from build123d import *

# Parameters (mm, degrees)
SKETCH_1_W      = 15.44
SKETCH_1_H      = 15.44
EXTRUDE_1_DEPTH = 17.2
SKETCH_3_R      = 4.9
EXTRUDE_2_DEPTH = 5.5
SKETCH_4_R      = 3.45
EXTRUDE_3_DEPTH = 2


with BuildPart() as part:
    # Эскиз1 → Бобышка-Вытянуть1 (new body)
    with BuildSketch(Plane(origin=(0, 0, 0), x_dir=(1, 0, 0), z_dir=(0, 1, 0))):
        Rectangle(SKETCH_1_W, SKETCH_1_H)
    extrude(amount=EXTRUDE_1_DEPTH)

    # Эскиз2 → section 0 of loft_1
    with BuildSketch(Plane(origin=(0, 29.9, 0), x_dir=(1, 0, 0), z_dir=(0, 1, 0)), mode=Mode.PRIVATE) as loft_1_s0:
        with BuildLine():
            Line((-5.5, 5.5), (5.5, 5.5))
            Line((5.5, 5.5), (5.5, -5.5))
            Line((5.5, -5.5), (-5.5, -5.5))
            Line((-5.5, -5.5), (-5.5, 5.5))
        make_face()
    # loft up to a face of the part (loft_1)
    loft([loft_1_s0.sketch, part.faces().sort_by_distance((0, 17.2, 0))[0]])

    # Эскиз3 → Бобышка-Вытянуть2 (add)
    with BuildSketch(Plane(origin=(0, 29.9, 0), x_dir=(1, 0, 0), z_dir=(0, 1, 0))):
        with Locations(Location((0, 0, 0), (0, 0, 270))):
            Circle(SKETCH_3_R)
    extrude(amount=EXTRUDE_2_DEPTH)

    # Эскиз4 → Бобышка-Вытянуть3 (add)
    with BuildSketch(Plane(origin=(0, 35.4, 0), x_dir=(1, 0, 0), z_dir=(0, 1, 0))):
        with Locations(Location((0, 0, 0), (0, 0, 270))):
            Circle(SKETCH_4_R)
    extrude(amount=EXTRUDE_3_DEPTH)


solid = part.part
Could you check a few things on this model? Use its own coordinates, in mm. A direction names the side the tool comes from. Round coordinates to 2 decimals unless told otherwise and drop trailing zeros.
(1) I'm going to push flat-ended pins straight in: pin 1 (3 mm diameter, centred on x = -2, y = 30, fed in from +Z); pin 2 (5 mm diameter, centred on y = 31.5, z = 2, fed in from +X); pin 3 (1 mm diameter, centred on x = 1, y = 32, fed in from -Z). Where does each tip first touch, or does it pass through?
Response values:
pin 1: stops at z = 5.74
pin 2: stops at x = 5.66
pin 3: stops at z = -4.87
(2) Please list where these lines run through material, in increasing order: line 1 along Y through (x, z) = (1.25, 3.5); line 2 along X through (y, z) = (19, -4.75); line 3 along X through (y, z) = (20, 1.25).
Response values:
line 1: y = 0 to 35.4
line 2: x = -7.41 to 7.41
line 3: x = -7.23 to 7.23
(3) Which directions (+Z, -Z, +X, -X, +Y, -Y) give clear straight access to the entire face, cutting with the end or side of a thin tool? Please do faces 1 (the flat face through (0, 8, -7.72)), 2 (the flat face through (-3, 35.4, 2)).
Response values:
face 1: -Z, +X, -X, +Y, -Y
face 2: +Y
